Source: CAD feature listing. Evaluate the final solid. Frame: model axes, mm. Round coordinates to 2 decimals unless told otherwise and drop trailing zeros. Loops run counter-clockwise (first coordinate to the right, second up) from the corner with the lowest first, then second, coordinate; pieces in that order, holes last.
Item 1: Section query C-C on y = -5. Return loops of the section in (x, z).
Item 2: Ray query, L1, parallel to X at y = -4, z = 7.5; L2, parallel to Z at x = 33, y = -0.25; L3, parallel to Z at x = -5.5, y = -5.25. Return the intervals inside material, ascending.
Item 3: Pull-direction query (Z, two-part tool) for faces 1 (the cylindrical face through (-0.99, -3.13, -152.49)), 2 (the flat face through (1, -6.35, -24)), 3 (the cylindrical face through (37.63, -3.22, 97.84)), 4 (the flat face through (1, -3, 107.5)); classes: released by +Z, released by -Z, zero draft, split by the parting line, or undercut.
Item 4: Section query A-A on z = 97.5. Return loops of the section in (x, y).
Item 5: Section query D-D on x = 35. Return loops of the section in (y, z), then the cut area to 3 significant figures.
Item 6: First-contact query: P1, Ø22.5, axis at x = 0, z = -107.5, coming from the +Y side. Flat tip, straight axial feed; report the tip coordinate or a pass-through.
Item 7: Section query B-B on x = 0. Return loops of the section in (y, z), then the cut area to 3 significant figures.
```python
from build123d import *

# Parameters (mm, degrees)
SKETCH1_R            = 12.5
BOSS_EXTRUDE1_DEPTH  = 6.35
M5_CLEARANCE_HOLE1_D = 5.3


with BuildPart() as part:
    # Sketch1 → Boss-Extrude1 (new body)
    with BuildSketch(Plane(origin=(0, 0, 0), x_dir=(1, 0, 0), z_dir=(0, 1, 0))):
        with BuildLine():
            Line((-45, -107.5), (-45, 107.5))
            ThreePointArc((-45, 107.5), (0, 152.5), (45, 107.5))
            Line((45, 107.5), (45, -107.5))
            Line((45, -107.5), (-45, -107.5))
        make_face()
        with Locations(Location((0, 107.5, 0), (0, 0, 270))):
            Circle(SKETCH1_R, mode=Mode.SUBTRACT)
    extrude(amount=-BOSS_EXTRUDE1_DEPTH)

    # M5 Clearance Hole1 (through all)
    with Locations(Plane(origin=(-35, 0, 7.5), x_dir=(0, 0, 1), z_dir=(0, 1, 0))):
        with Locations((0, 0), (0, 70), (90, 0), (90, 70)):
            Hole(M5_CLEARANCE_HOLE1_D / 2)


solid = part.part
```
Data:
1. outline: (-45, -107.5) arc R45 ccw to (45, -107.5) - (45, 107.5) - (-45, 107.5) - close; hole circle Ø5.3 at (-35, 7.5); hole circle Ø5.3 at (-35, 97.5); hole circle Ø25 at (0, -107.5); hole circle Ø5.3 at (35, 7.5); hole circle Ø5.3 at (35, 97.5)
2. L1: x = -45 to -37.65, -32.35 to 32.35, 37.65 to 45
2. L2: z = -138.09 to 5.76, 9.24 to 95.76, 99.24 to 107.5
2. L3: z = -152.16 to -118.72, -96.28 to 107.5
3. face 1: released by -Z
3. face 2: zero draft
3. face 3: undercut
3. face 4: released by +Z
4. outline: (-45, -6.35) - (-37.65, -6.35) - (-37.65, 0) - (-45, 0) - close; (-32.35, -6.35) - (32.35, -6.35) - (32.35, 0) - (-32.35, 0) - close; (37.65, -6.35) - (45, -6.35) - (45, 0) - (37.65, 0) - close
5. outline: (-6.35, -135.78) - (0, -135.78) - (0, 4.85) - (-6.35, 4.85) - close; (-6.35, 10.15) - (0, 10.15) - (0, 94.85) - (-6.35, 94.85) - close; (-6.35, 100.15) - (0, 100.15) - (0, 107.5) - (-6.35, 107.5) - close
5. area: 1,480 mm2
6. P1: passes through
7. outline: (-6.35, -152.5) - (0, -152.5) - (0, -120) - (-6.35, -120) - close; (-6.35, -95) - (0, -95) - (0, 107.5) - (-6.35, 107.5) - close
7. area: 1,490 mm2
